Design review of the part built by this model. Coordinates are the model's own, in mm. A direction names the side the tool comes from. Coordinates: 2 decimals unless noted, no trailing zeros. Loops run counter-clockwise (first coordinate to the right, second up) from the corner with the lowest first, then second, coordinate; pieces in that order, holes last. Notation, with made-up numbers: M -4,23 L 7,23 A14 cw 7,29 Z; hole C 82,54.25 d2. An arc over 180 degrees is marked long. Answer as a JSON object with one key per item and string values. Group by question number.
1. Draft analysis for pull direction Z (two halves, no side actions). For faces 3 (the cylindrical face through (-34.287, 4.248, -0.046)), 4 (the flat face through (-30, 2, 0)), 5 (the flat face through (30, 2, 0)), 6 (the cylindrical face through (0.455, 0.752, 5.037)), state which applies: +Z half, -Z half, draft (parallel to the pull), parting line (faces both ways), or undercut.
2. Insertion check: pin 1 (6 mm diameter, centred on x = 19, z = 0, fed in from -Y); pin 2 (0.8 mm diameter, centred on y = 1.5, z = 0, fed in from -X). Each pin has a flat end and moves straight along its axis. Give the tip position at first contact, or say it passes through.
3. Machinability: for faces 1 (the flat face through (0, 2, 0.75)), 2 (the cylindrical face through (34.287, 0.752, -0.046)), which of the approach directions +Z, -Z, +X, -X, +Y, -Y give a long, thin tool a straight path to every point of the face, cutting with its end or side? Answer none if there is none.
4. Consider section C-C (y = 4.05). State the section outline as (x, z) points, then the cut area to 3 significant figures.
5. To check wall thickness, follow probe 1 along Z at (x, y) = (1, 1.5); probe 2 along Z at (x, y) = (-3, 0.55); probe 3 along X at (y, z) = (2.4, -2). State the ranges of each line that lie inside material, in increasing order.
from build123d import *

# Parameters (mm, degrees)
ESQUISSE4_W        = 70
ESQUISSE4_H        = 11.5
ESQUISSE4_W_2      = 60
ESQUISSE4_H_2      = 1.5
BOSS_EXTRU_2_DEPTH = 5
CONG_1_R           = 2.5


with BuildPart() as part:
    # Esquisse4 → Boss.-Extru.2 (new body)
    with BuildSketch(Plane(origin=(0, 0, 0), x_dir=(1, 0, 0), z_dir=(0, 1, 0))):
        Rectangle(ESQUISSE4_W, ESQUISSE4_H)
        Rectangle(ESQUISSE4_W_2, ESQUISSE4_H_2, mode=Mode.SUBTRACT)
    extrude(amount=BOSS_EXTRU_2_DEPTH)

    # Congé1
    cong_1_edges = [part.edges().sort_by_distance(p)[0] for p in [
        (-35, 5, 0),
        (0, 5, 5.75),
        (35, 5, 0),
        (0, 0, 5.75),
        (-35, 0, 0),
        (0, 0, -5.75),
        (35, 0, 0),
        (0, 5, -5.75),
        (35, 2.5, 5.75),
        (-35, 2.5, 5.75),
        (-35, 2.5, -5.75),
        (35, 2.5, -5.75),
    ]]
    fillet(cong_1_edges, radius=CONG_1_R - 0.0001)  # a hair under: the kernel refuses the full size


solid = part.part
Findings below:
{
 "1": {"face 3": "draft", "face 4": "undercut", "face 5": "undercut", "face 6": "+Z half"},
 "2": {"pin 1": "stops at y = 0", "pin 2": "stops at x = -34.93"},
 "3": {"face 1": "+Y, -Y", "face 2": "+Z, -Z, +X, -Y"},
 "4": {"outline": "M -34.46,-3.25 A1.96 ccw -32.5,-5.21 L 32.5,-5.21 A1.96 ccw 34.46,-3.25 L 34.46,3.25 A1.96 ccw 32.5,5.21 L -32.5,5.21 A1.96 ccw -34.46,3.25 Z; hole M -30,-0.75 L 30,-0.75 L 30,0.75 L -30,0.75 Z", "area": "625 mm^2"},
 "5": {"probe 1": "z = -5.54 to -0.75, 0.75 to 5.54", "probe 2": "z = -4.81 to -0.75, 0.75 to 4.81", "probe 3": "x = -35 to 35"}
}
